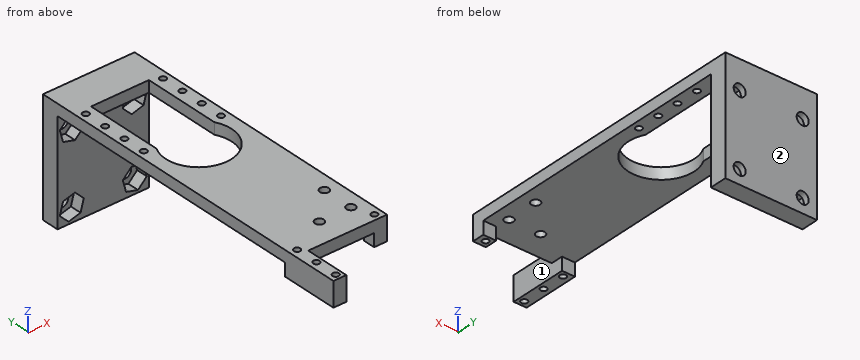
Autodesk Inventor part; units mm, degrees
ref_plane "YZ Plane" through (0, 0, 0) normal (1, 0, 0) x (0, 1, 0)
ref_plane "XZ Plane" through (0, 0, 0) normal (0, 1, 0) x (-1, 0, 0)
ref_plane "Plan de construction4" through (0, 0, 21) normal (0, 0, 1) x (1, 0, 0)
sketch "Esquisse" plane through (0, 0, 21) normal (0, 0, 1) x (1, 0, 0)
  circle A0 centre (0, 0) radius 11.5
  line L0 (16, -11.5) -> (-16, -11.5) construction
  line L1 (-16, -11.5) -> (-16, 38.5)
  line L2 (-16, 38.5) -> (16, 38.5)
  line L3 (16, 38.5) -> (16, -11.5)
  line L4 (0, 0) -> (-13.5, 6.75) construction
  circle A1 centre (-13.5, 6.75) radius 1.1
  line L5 (-13.5, 6.75) -> (-13.5, 14.75) construction
  line L6 (-13.5, 14.75) -> (-13.5, 22.75) construction
  line L7 (-13.5, 22.75) -> (-13.5, 30.75) construction
  circle A2 centre (-13.5, 30.75) radius 1.1
  circle A3 centre (-13.5, 22.75) radius 1.1
  circle A4 centre (-13.5, 14.75) radius 1.1
  line L8 (-22.4, 0) -> (22.4, 0) construction
  line L9 (10.1, 32.6) -> (10.1, 5.4991)
  line L10 (-10.1, 5.4991) -> (-10.1, 32.6)
  line L11 (-10.1, 32.6) -> (10.1, 32.6)
  line L12 (16, -11.5) -> (0, 0) construction
  line L13 (-16, -11.5) -> (0, 0) construction
  line L14 (10.1, 5.4991) -> (-10.1, 5.4991) construction
  line L15 (16, 38.5) -> (-16, 38.5)
  line L16 (-16, 38.5) -> (-16, 39.5)
  line L17 (-16, 39.5) -> (16, 39.5)
  line L18 (16, 39.5) -> (16, 38.5)
  line L19 (0, -98.8) -> (0, 69.55) construction
  circle A5 centre (13.5, 6.75) radius 1.1
  circle A6 centre (13.5, 30.75) radius 1.1
  circle A7 centre (13.5, 22.75) radius 1.1
  circle A8 centre (13.5, 14.75) radius 1.1
  line L20 (-16, -11.5) -> (16, -11.5) construction
  line L21 (16, -11.5) -> (16, -16.5)
  line L22 (16, -16.5) -> (-16, -16.5)
  line L23 (-16, -16.5) -> (-16, -11.5)
  line L24 (16, 39.5) -> (-16, 39.5)
  line L25 (-16, 39.5) -> (-16, 45.5)
  line L26 (-16, 45.5) -> (16, 45.5)
  line L27 (16, 45.5) -> (16, 39.5)
  line L28 (16, -16.5) -> (-16, -16.5)
  line L29 (-16, -16.5) -> (-16, -59)
  line L30 (-16, -59) -> (-11.5, -59)
  line L31 (16, -59) -> (16, -16.5)
  circle A9 centre (0, -50) radius 1.55
  line L32 (13.5, -56.75) -> (-13.5, -56.75) construction
  line L33 (-13.5, -56.75) -> (-13.5, -64.75) construction
  line L34 (-13.5, -64.75) -> (-13.5, -72.75) construction
  line L35 (-13.5, -72.75) -> (13.5, -72.75) construction
  line L36 (13.5, -72.75) -> (13.5, -64.75) construction
  line L37 (13.5, -64.75) -> (13.5, -56.75) construction
  circle A10 centre (13.5, -72.75) radius 1.1
  circle A11 centre (13.5, -64.75) radius 1.1
  circle A12 centre (13.5, -56.75) radius 1.1
  circle A13 centre (-13.5, -56.75) radius 1.1
  circle A14 centre (-13.5, -64.75) radius 1.1
  circle A15 centre (-13.5, -72.75) radius 1.1
  line L38 (16, -54.75) -> (11.5, -54.75)
  line L39 (11.5, -54.75) -> (11.5, -59)
  line L40 (-11.5, -59) -> (-11.5, -54.75)
  line L41 (-11.5, -54.75) -> (-16, -54.75)
  line L42 (-11.5, -59) -> (16, -59)
  line L43 (-11.5, -59) -> (-11.5, -74.75)
  line L44 (-11.5, -74.75) -> (-16, -74.75)
  line L45 (-16, -74.75) -> (-16, -59)
  line L46 (0, -50) -> (11, -50) construction
  line L47 (11, -50) -> (11, -39) construction
  circle A16 centre (11, -50) radius 1.55
  circle A17 centre (11, -39) radius 1.55
  point P0 (0, -11.5)
  point P1 (16, -11.5)
  dimension "d107" = 23
  dimension "d133" = 6.75
  dimension "d135" = 2.2
  dimension "d137" = 8
  dimension "d138" = 20.2
  dimension "d160" = 50
  dimension "d161" = 5.9
  dimension "d162" = 32
  dimension "d163" = 11.5
  dimension "d169" = 5
  dimension "d224" = 1
  dimension "d225" = 6
  dimension "d240" = 13.5
  dimension "d242" = 32
  dimension "d243" = 3.1
  dimension "d249" = 50
  dimension "d250" = 6.75
  dimension "d251" = 8
  dimension "d252" = 2.2
  dimension "d253" = 2
  dimension "d254" = 2
  dimension "d255" = 9
  dimension "d258" = 2
  dimension "d261" = 3.1
  dimension "d263" = 11
  dimension "d264" = 11
extrude "Face fixation moteur" add sketch "Esquisse" against normal blind 4 contours L1 L2 L3 L21 L22 L23 | L16 L17 L18 L2 | L22 L31 L38 L39 L42 L40 L41 L29 | L41 L40 L30 L29 | L31 L42 L39 L38
extrude "Creux moteur" [suppressed]
extrude "Rai basl" add sketch "Esquisse" against normal blind 40 contours L25 L26 L27 L17
sketch "Esquisse16" plane through (-16, 39.5, 17) normal (0, -1, 0) x (1, 0, 0)
  line L0 (0, 0) -> (0, -36)
  line L1 (32, -36) -> (0, -36)
  line L2 (32, 0) -> (32, -36)
  line L3 (5, -6) -> (27, -6) construction
  line L4 (27, -6) -> (27, -31) construction
  line L5 (27, -31) -> (5, -31) construction
  line L6 (5, -31) -> (5, -6) construction
  line L7 (0, 0) -> (0, -36)
  line L8 (0, -1) -> (5, -6) construction
  line L9 (5, -31) -> (0, -36) construction
  line L10 (0, -36) -> (32, -36)
  line L11 (27, -31) -> (32, -36) construction
  circle A0 centre (5, -6) radius 2.1
  circle A1 centre (27, -6) radius 2.1
  circle A2 centre (27, -31) radius 2.1
  circle A3 centre (5, -31) radius 2.1
  line L12 (6.1207, -10.1826) -> (1.9381, -9.0619)
  line L13 (1.9381, -9.0619) -> (0.8174, -4.8793)
  line L14 (0.8174, -4.8793) -> (3.8793, -1.8174)
  line L15 (3.8793, -1.8174) -> (8.0619, -2.9381)
  line L16 (8.0619, -2.9381) -> (9.1826, -7.1207)
  line L17 (9.1826, -7.1207) -> (6.1207, -10.1826)
  line L18 (9.1826, -29.8793) -> (8.0619, -34.0619)
  line L19 (8.0619, -34.0619) -> (3.8793, -35.1826)
  line L20 (3.8793, -35.1826) -> (0.8174, -32.1207)
  line L21 (0.8174, -32.1207) -> (1.9381, -27.9381)
  line L22 (1.9381, -27.9381) -> (6.1207, -26.8174)
  line L23 (6.1207, -26.8174) -> (9.1826, -29.8793)
  line L24 (25.8793, -26.8174) -> (30.0619, -27.9381)
  line L25 (30.0619, -27.9381) -> (31.1826, -32.1207)
  line L26 (31.1826, -32.1207) -> (28.1207, -35.1826)
  line L27 (28.1207, -35.1826) -> (23.9381, -34.0619)
  line L28 (23.9381, -34.0619) -> (22.8174, -29.8793)
  line L29 (22.8174, -29.8793) -> (25.8793, -26.8174)
  line L30 (22.8174, -7.1207) -> (23.9381, -2.9381)
  line L31 (23.9381, -2.9381) -> (28.1207, -1.8174)
  line L32 (28.1207, -1.8174) -> (31.1826, -4.8793)
  line L33 (31.1826, -4.8793) -> (30.0619, -9.0619)
  line L34 (30.0619, -9.0619) -> (25.8793, -10.1826)
  line L35 (25.8793, -10.1826) -> (22.8174, -7.1207)
  line L36 (7.6517, -8.6517) -> (24.3483, -8.6517) construction
  line L37 (24.3483, -8.6517) -> (24.3483, -28.3483) construction
  line L38 (24.3483, -28.3483) -> (7.6517, -28.3483) construction
  line L39 (7.6517, -28.3483) -> (7.6517, -8.6517) construction
  line L40 (32, 4) -> (0, 4)
  line L41 (26.1, 4) -> (5.9, 4)
  line L42 (5.9, 4) -> (26.1, 4)
  line L43 (28.4, 4) -> (30.6, 4)
  line L44 (28.4, 4) -> (30.6, 4)
  line L45 (1.4, 4) -> (3.6, 4)
  line L46 (1.4, 4) -> (3.6, 4)
  line L47 (1.4, 4) -> (3.6, 4)
  line L48 (1.4, 4) -> (3.6, 4)
  line L49 (28.4, 4) -> (30.6, 4)
  line L50 (28.4, 4) -> (30.6, 4)
  line L51 (32, 0) -> (32, -36)
  line L52 (0, 0) -> (0, -36)
  line L53 (32, -1) -> (27, -6) construction
  line L54 (0, -1) -> (32, -1)
  line L55 (0, 0) -> (32, 0)
  line L56 (0, 4) -> (32, 4)
  point P0 (16, -17)
  dimension "d228" = 5
  dimension "d229" = 5
  dimension "d230" = 4.2
  dimension "d231" = 7.5
  dimension "d232" = 25
  dimension "d233" = 22
  dimension "d245" = 40
  dimension "d246" = 32
  dimension "d248" = 1
extrude "Extrusion23" cut sketch "Esquisse16" against normal through all contours A0 | A1 | A2 | A3
extrude "Extrusion24" cut sketch "Esquisse16" against normal blind 4 contours A3 | L12 L13 L14 L15 L16 L17 | L18 L19 L20 L21 L22 L23 | L24 L25 L26 L27 L28 L29 | L30 L31 L32 L33 L34 L35
extrude "Extrusion25" add sketch "Esquisse" against normal blind 8.5 contours L41 L40 L30 L29 | L31 L42 L39 L38 | L30 L43 L44 L45
properties part number "Support AX 12A"
Here's how the part is built. I have some questions about the finished solid (model axes, mm). Face numbers are marked on the shaded views. A direction names the side the tool comes from. Coordinates: 2 decimals unless noted, no trailing zeros. Write each loop counter-clockwise with the first axis right and the second up, starting at its lowest first coordinate (ties: lowest second). Pieces come first, ordered by that corner, then holes.
1) If we section it at C-C (z = 19): Count the separate pieces of the cut face and the enclosed holes in it, plus the area to 3 significant figures.
Filled in:
separate pieces: 1
enclosed holes: 16
area: 2,470 mm2
2) If I drill on line 1 (Y direction, x = 0, z = 18.45); line 2 (Z direction, x = 11, y = 44.85); line 3 (Y direction, x = 13.5, z = 15.75), over which ranges is the centre line in solid material (lowest first)?
Filled in:
line 1: y = -59 to -51.55, -48.45 to -11.5, 32.6 to 45.5
line 2: z = -19 to -16.1, -11.9 to 8.9, 13.1 to 21
line 3: y = -59 to -57.85, -55.65 to -54.75, 39.5 to 45.5
3) If we section it at B-B (y = 0): List the corners of the cut face in (x, z) for me.
Filled in:
outline: (-16, 17) - (-11.5, 17) - (-11.5, 21) - (-16, 21) - close; (11.5, 17) - (16, 17) - (16, 21) - (11.5, 21) - close
4) Which directions (+Z, -Z, +X, -X, +Y, -Y) give clear straight access to the entire face, cutting with the end or side of a thin tool? Please do the marked faces 1 and 2.
Filled in:
face 1: -Z, -Y
face 2: +Z, -Z, +X, -X, +Y
5) If we section it at A-A (y = -50): List the corners of the cut face in (x, z) for me.
Filled in:
outline: (-16, 17) - (-1.55, 17) - (-1.55, 21) - (-16, 21) - close; (1.55, 17) - (9.45, 17) - (9.45, 21) - (1.55, 21) - close; (12.55, 17) - (16, 17) - (16, 21) - (12.55, 21) - close
6) If we section it at D-D (z = -14): List the corners of the cut face in (x, y) for me.
Filled in:
outline: (-16, 39.5) - (-14.88, 39.5) - (-14.88, 43.5) - (-13.1, 43.5) - (-13.1, 45.5) - (-16, 45.5) - close; (-8.9, 43.5) - (-7.12, 43.5) - (-7.12, 39.5) - (7.12, 39.5) - (7.12, 43.5) - (8.9, 43.5) - (8.9, 45.5) - (-8.9, 45.5) - close; (13.1, 43.5) - (14.88, 43.5) - (14.88, 39.5) - (16, 39.5) - (16, 45.5) - (13.1, 45.5) - close
7) I'm going to push flat-ended pins straight in: pin 1 (4 mm diameter, centred on x = 12.5, z = 9.5, fed in from -Y); pin 2 (1.3 mm diameter, centred on x = -13.5, y = -64.75, fed in from -Z); pin 3 (4 mm diameter, centred on x = 11, y = -50, fed in from -Z); pin 4 (4.5 mm diameter, centred on x = 5, z = 18.5, fed in from -Y). Where does each tip first touch, or does it pass through?
Filled in:
pin 1: stops at y = 39.5
pin 2: passes through
pin 3: stops at z = 17
pin 4: stops at y = -59
